Verification items for the finished model (mm, model axes). Give positions to 0.01 mm unless a question says otherwise; leave off trailing zeros. Write each loop counter-clockwise with the first axis right and the second up, starting at its lowest first coordinate (ties: lowest second). Pieces come first, ordered by that corner, then holes. Notation, with made-up numbers: (15.25, 65) -> (69.25, 65) arc R16 cw to (69.25, 76) -> close; hole circle Ø2 at (-9.75, -16). An arc over 180 degrees is marked (long way). Use one line per item in the form item = value. Start each with the question number.
(1) Section check B-B, the plane z = 1.75. State how many separate pieces and enclosed holes the cut face has, plus the area to 3 significant figures.
(2) Scan lines: L1, parallel to X at y = 194, z = 1.5; L2, parallel to X at y = 174.5, z = 1.15; L3, parallel to Y at x = 434, z = 1.85. Record each from-to range of solid material in increasing order.
(3) Depth check by flat-ended pin: pin 1 Ø2.5 at (y, z) = (198.5, 2) entering from -X; pin 2 Ø3 at (x, y) = (252.5, 174.5) entering from -Z; pin 3 Ø2.5 at (y, z) = (193.5, 2) entering from +X; pin 4 Ø2.5 at (x, z) = (482, 2) entering from +Y. Enter the tip coordinate at first touch or a pass-through.
(4) Section check A-A, the plane x = 174. Record the cut outline in (y, z), plus the area to 3 significant figures.
from build123d import *

# Parameters (mm, degrees)
SKETCH1_W           = 7.5
SKETCH1_H           = 5
SKETCH1_W_2         = 10
BOSS_EXTRUDE1_DEPTH = 5


with BuildPart() as part:
    # Sketch1 → Boss-Extrude1 (new body)
    with BuildSketch(Plane.XY):
        Polygon((480, 177.5), (485, 177.5), (485, 187.5), (480, 187.5), (480, 190), (472.5, 190), (472.5, 195), (480, 195), (480, 200), (447.5, 200), (447.5, 195), (377.5, 195), (377.5, 200), (337.5, 200), (337.5, 195), (305, 195), (305, 190), (295, 190), (295, 195), (280, 195), (280, 190), (270, 190), (270, 195), (217.5, 195), (217.5, 200), (177.5, 200), (177.5, 195), (107.5, 195), (107.5, 200), (75, 200), (75, 195), (75, 187.5), (70, 187.5), (70, 177.5), (75, 177.5), (75, 170), (480, 170), align=None)
        with Locations((453.75, 192.5)):
            Rectangle(SKETCH1_W, SKETCH1_H, mode=Mode.SUBTRACT)
        with Locations((95, 192.5)):
            Rectangle(SKETCH1_W_2, SKETCH1_H, mode=Mode.SUBTRACT)
    extrude(amount=BOSS_EXTRUDE1_DEPTH)


solid = part.part
Completed:
q1.separate_pieces = 1
q1.enclosed_holes = 2
q1.area = 10,700 mm²
q2.L1 = 75 to 90, 100 to 270, 280 to 295, 305 to 450, 457.5 to 472.5
q2.L2 = 75 to 480
q2.L3 = 170 to 195
q3.pin_1 = 75
q3.pin_2 = 0
q3.pin_3 = 472.5
q3.pin_4 = 187.5
q4.outline = (170, 0) -> (195, 0) -> (195, 5) -> (170, 5) -> close
q4.area = 125 mm²
